Autodesk Inventor part; units mm, degrees
ref_plane "YZ Plane" through (0, 0, 0) normal (1, 0, 0) x (0, 1, 0)
ref_plane "XZ Plane" through (0, 0, 0) normal (0, 1, 0) x (-1, 0, 0)
ref_plane "XY Plane" through (0, 0, 0) normal (0, 0, 1) x (1, 0, 0)
sketch "Sketch1" plane through (0, 0, 0) normal (0, 0, 1) x (1, 0, 0)
  line L0 (0, 0) -> (44.45, 0)
  line L1 (44.45, 0) -> (44.45, 22.86)
  line L2 (44.45, 22.86) -> (0, 22.86)
  line L3 (0, 22.86) -> (0, 0)
  dimension "d0" = 22.86
  dimension "d1" = 44.45
extrude "Extrusion1" add sketch "Sketch1" along normal blind 2.54
sketch "Sketch2" plane through (0, 0, 2.54) normal (0, 0, 1) x (1, 0, 0)
  line L0 (0, 0) -> (44.45, 0)
  line L1 (44.45, 22.86) -> (41.91, 22.86)
  line L2 (41.91, 22.86) -> (41.91, 0)
  line L3 (41.91, 0) -> (44.45, 0)
  line L4 (44.45, 0) -> (44.45, 22.86)
  dimension "d4" = 2.54
extrude "Extrusion2" add sketch "Sketch2" along normal blind 35.56
sketch "Sketch4" plane through (0, 0, 2.54) normal (0, 0, 1) x (1, 0, 0)
  line L0 (-11.3987, 11.43) -> (43.7828, 11.43) construction
  line L1 (0, 0) -> (41.91, 0) construction
  line L2 (41.91, 0) -> (41.91, 22.86) construction
  line L3 (41.91, 22.86) -> (0, 22.86) construction
  line L4 (0, 22.86) -> (0, 0) construction
  line L5 (0, 0) -> (41.91, 0) construction
  point P0 (15.24, 11.43)
  dimension "d16" = 11.43
  dimension "d17" = 26.67
hole "Hole2" at (15.24, 11.43, 2.54) direction (0, 0, -1) diameter 3.2512 end through all
sketch "Sketch5" plane through (41.91, 0, 2.54) normal (-1, 0, 0) x (0, 0, 1)
  line L0 (24.13, 11.4617) -> (25.4, 11.4617)
  circle A0 centre (25.4, 11.4617) radius 1.6412
  line L1 (0, 0) -> (0, 22.86)
  point P0 (-2.54, 0)
  dimension "d25" = 1.27
  dimension "d28" = 25.4
extrude "Extrusion3" cut sketch "Sketch5" against normal blind 25.4
properties part number "000102 (revised)"
CAD build for the part. Positions are in the model's coordinates, mm. A direction names the side the tool comes from. Round coordinates to 2 decimals unless told otherwise and drop trailing zeros. Order: outer loops, then holes, each group sorted by start corner. A loop starts at its lowest first (then second) coordinate and runs counter-clockwise, first axis right, second up.
Item 1: Saw through at B-B on z = 27.94. Write the cut outline in (x, y).
Item 2: Tool access for faces 4 (the face through (44.45, 11, 19)), 5 (the face through (41.91, 12, 20)): list every direction of +Z, -Z, +X, -X, +Y, -Y with a clear straight run to the whole face (end or side of a thin tool).
Item 3: Pin check, flat tips, straight feed: pin 1 (7 mm diameter, centred on y = 8, z = 29, fed in from -X); pin 2 (7 mm diameter, centred on x = 19.5, y = 12, fed in from +Z); pin 3 (5 mm diameter, centred on x = 8, y = 15.5, fed in from -Z). Stop position of each tip, or through.
Item 4: Saw through at A-A on x = 15.24. Write the cut outline in (y, z).
Item 5: Probe line 1 along Y through (x, z) = (43.7, 27.94); line 2 along X through (y, z) = (11.43, 0.95); line 3 along Z through (x, y) = (26.5, 6.75). List the from-to ranges inside material, lowest first.
Item 6: Mould opens along Z. For faces 1 (the face through (43.16, 12.57, 26.73)), 2 (the face through (22, 12, 0)), 3 (the face through (15.863, 9.928, 1.252)) say: pulls with the +Z half, pulls with the -Z half, needs draft (parallel to the pull), parting line crosses it, or undercut.
Item 7: Saw through at C-C on y = 2.75. Write the cut outline in (x, z), then the cut area to 3 significant figures.
Item 8: Saw through at D-D on x = 35.5. Write the cut outline in (y, z), then the cut area to 3 significant figures.
Reported:
1. outline: (41.91, 0) - (44.45, 0) - (44.45, 9.82) - (41.91, 9.82) - close; (41.91, 13.1) - (44.45, 13.1) - (44.45, 22.86) - (41.91, 22.86) - close
2. face 4: +Z, -Z, +X, +Y, -Y
2. face 5: +Z, -X, +Y, -Y
3. pin 1: stops at x = 41.91
3. pin 2: stops at z = 2.54
3. pin 3: stops at z = 0
4. outline: (0, 0) - (9.8, 0) - (9.8, 2.54) - (0, 2.54) - close; (13.06, 0) - (22.86, 0) - (22.86, 2.54) - (13.06, 2.54) - close
5. line 1: y = 0 to 9.82, 13.1 to 22.86
5. line 2: x = 0 to 13.61, 16.87 to 44.45
5. line 3: z = 0 to 2.54
6. face 1: undercut
6. face 2: pulls with the -Z half
6. face 3: needs draft
7. outline: (0, 0) - (44.45, 0) - (44.45, 38.1) - (41.91, 38.1) - (41.91, 2.54) - (0, 2.54) - close
7. area: 203 mm2
8. outline: (0, 0) - (22.86, 0) - (22.86, 2.54) - (0, 2.54) - close
8. area: 58.1 mm2
